from build123d import *

# Parameters (mm, degrees)
BOSS_EXTRUDE1_DEPTH = 12.7
SKETCH3_W           = 13.716
SKETCH3_H           = 15.24
CUT_EXTRUDE1_DEPTH  = 12.7
SKETCH4_R           = 2.54
SKETCH4_R_2         = 3.81
CUT_EXTRUDE2_DEPTH  = 91.44
SKETCH7_W           = 22.86
SKETCH7_H           = 30.48
CUT_EXTRUDE10_DEPTH = 18.288
SKETCH8_R           = 5.08
CUT_EXTRUDE12_DEPTH = 54.61


with BuildPart() as part:
    # Sketch1 → Boss-Extrude1 (new body)
    with BuildSketch(Plane(origin=(0, 0, 0), x_dir=(1, 0, 0), z_dir=(0, 1, 0))):
        Polygon((63.5, 0), (88.9, 0), (88.9, 101.6), (0, 101.6), (0, 0), (38.1, 0), (38.1, -25.4), (63.5, -25.4), align=None)
    extrude(amount=BOSS_EXTRUDE1_DEPTH)

    # Sketch3 → Cut-Extrude1 (cut)
    with BuildSketch(Plane(origin=(0, 12.7, 0), x_dir=(1, 0, 0), z_dir=(0, 1, 0))):
        with Locations((18.858, 93.98)):
            Rectangle(SKETCH3_W, SKETCH3_H)
        with Locations((44.512, 93.98)):
            Rectangle(SKETCH3_W, SKETCH3_H)
        with Locations((70.166, 93.98)):
            Rectangle(SKETCH3_W, SKETCH3_H)
    extrude(amount=-CUT_EXTRUDE1_DEPTH, mode=Mode.SUBTRACT)

    # Sketch4 → Cut-Extrude2 (cut)
    with BuildSketch(Plane.ZY):
        with Locations((-93.98, 6.35)):
            Circle(SKETCH4_R)
        with Locations((12.7, 6.35)):
            Circle(SKETCH4_R_2)
    extrude(amount=-CUT_EXTRUDE2_DEPTH, mode=Mode.SUBTRACT)

    # Sketch7 → Cut-Extrude10 (cut)
    with BuildSketch(Plane.XZ):
        with Locations((11.43, -28.172925588)):
            Rectangle(SKETCH7_W, SKETCH7_H)
    extrude(amount=-CUT_EXTRUDE10_DEPTH, mode=Mode.SUBTRACT)

    # Sketch8 → Cut-Extrude12 (cut)
    with BuildSketch(Plane.XY):
        with Locations((11.43, 6.168740828)):
            Circle(SKETCH8_R)
    extrude(amount=-CUT_EXTRUDE12_DEPTH, mode=Mode.SUBTRACT)


solid = part.part
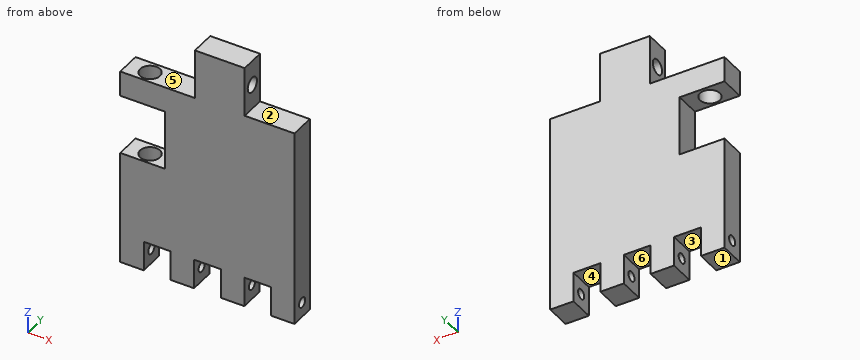
Could you check a few things on this model? Use its own coordinates, in mm. Face numbers are marked on the shaded views. A direction names the side the tool comes from. Round coordinates to 2 decimals unless told otherwise and drop trailing zeros. Write each loop counter-clockwise with the first axis right and the second up, starting at its lowest first coordinate (ties: lowest second). Pieces come first, ordered by that corner, then holes. Notation, with made-up numbers: (50, -7) - (104, -7) arc R20 cw to (104, 10) - close; hole circle Ø6 at (-12, 67.25). An arc over 180 degrees is marked (long way). Use a Markdown table: item, result.
Q1. For the marked faces 1, 2 and 3, which set-ups out of +Z, -Z, +X, -X, +Y, -Y let a thin tool reach every point of the face, with its end or its side?
Output values:
| item | result |
|---|---|
| face 1 | -Z, +X, -X, +Y, -Y |
| face 2 | +Z, +X, +Y, -Y |
| face 3 | -Z, +Y, -Y |
Q2. I want a section at C-C (z = 12.7). List the corners of the cut face in (x, y) for me, plus the area to 3 significant figures.
Output values:
| item | result |
|---|---|
| outline | (38.1, 0) - (63.5, 0) - (63.5, 2.54) - (38.1, 2.54) - close; (38.1, 10.16) - (63.5, 10.16) - (63.5, 12.7) - (38.1, 12.7) - close |
| area | 129 mm2 |
Q3. For pin 1 (4 mm diameter, centred on y = 3.5, z = -29.5, fed in from -X); pin 2 (6.5 mm diameter, centred on x = 45.5, y = 3.5, fed in from -Z); pin 3 (6.5 mm diameter, centred on x = 23, y = 9, fed in from +Z), each with a flat end and sliding along its axis, tell me the tip position at first contact or that it passes through.
Output values:
| item | result |
|---|---|
| pin 1 | x = 22.86 |
| pin 2 | z = -86.36 |
| pin 3 | z = 0 |
Q4. I want a section at D-D (x = 49). List the corners of the cut face in (y, z) for me, plus the area to 3 significant figures.
Output values:
| item | result |
|---|---|
| outline | (0, -86.36) - (12.7, -86.36) - (12.7, 25.4) - (0, 25.4) - close; hole circle Ø7.62 at (6.35, 12.7) |
| area | 1,370 mm2 |
Q5. Thinking about a two-plate mould opening in X: for the marked faces 4, 5 and 6, which applies, released by +X, released by -X, zero draft, split by the parting line, or undercut?
Output values:
| item | result |
|---|---|
| face 4 | undercut |
| face 5 | zero draft |
| face 6 | undercut |
Q6. I want a section at A-A (x = 19.5). List the corners of the cut face in (y, z) for me, plus the area to 3 significant figures.
Output values:
| item | result |
|---|---|
| outline | (0, -86.36) - (12.7, -86.36) - (12.7, -43.41) - (0, -43.41) - close; (0, -12.93) - (12.7, -12.93) - (12.7, 0) - (0, 0) - close |
| area | 710 mm2 |
Q7. I want a section at B-B (z = -93.98). Count the separate pieces of the cut face and the enclosed holes in it, plus the area to 3 significant figures.
Output values:
| item | result |
|---|---|
| separate pieces | 8 |
| enclosed holes | 0 |
| area | 364 mm2 |
Q8. Please list where these lines run through material, in increasing order: L1, parallel to X at y = 2.5, z = -90.5; L2, parallel to Y at x = 11.43, z = -47; L3, parallel to Z at x = 17.5, y = 11.25.
Output values:
| item | result |
|---|---|
| L1 | 0 to 12, 25.72 to 37.65, 51.37 to 63.31, 77.02 to 88.9 |
| L2 | 0 to 1.09, 11.25 to 12.7 |
| L3 | -86.36 to -43.41, -12.93 to 0 |
